Build history of the part. All positions in model axes, mm. A direction names the side the tool comes from. Give positions to 0.01 mm unless a question says otherwise; leave off trailing zeros. Order: outer loops, then holes, each group sorted by start corner. A loop starts at its lowest first (then second) coordinate and runs counter-clockwise, first axis right, second up. Notation, with made-up numbers: (-27, -19) - (30, -19) arc R25 ccw to (30, 20) - close; hole circle Ø5 at (23, 38). An arc over 180 degrees is marked (long way). Answer in a Markdown table with one row per item.
```python
from build123d import *

# Parameters (mm, degrees)
SKETCH1_R           = 18.25
BOSS_EXTRUDE1_DEPTH = 57
SKETCH2_R           = 6.5
BOSS_EXTRUDE2_DEPTH = 5
FILLET1_R           = 1.5
SKETCH3_R           = 1.6
BOSS_EXTRUDE3_DEPTH = 8.5
BOSS_EXTRUDE4_START = -2.5
SKETCH4_R           = 3.9
BOSS_EXTRUDE4_DEPTH = 5
SKETCH5_R           = 5
BOSS_EXTRUDE5_DEPTH = 3
SKETCH6_R           = 1.5
BOSS_EXTRUDE6_DEPTH = 2
SKETCH7_W           = 0.5
SKETCH7_H           = 5
BOSS_EXTRUDE7_DEPTH = 10
CHAMFER1_SIZE       = 1


with BuildPart() as part:
    # Sketch1 → Boss-Extrude1 (new body)
    with BuildSketch(Plane(origin=(0, 0, 0), x_dir=(1, 0, 0), z_dir=(0, 1, 0))):
        Circle(SKETCH1_R)
    extrude(amount=BOSS_EXTRUDE1_DEPTH)

    # Sketch2 → Boss-Extrude2 (add)
    with BuildSketch(Plane(origin=(0, 57, 0), x_dir=(1, 0, 0), z_dir=(0, 1, 0))):
        Circle(SKETCH2_R)
    extrude(amount=BOSS_EXTRUDE2_DEPTH)

    # Fillet1
    fillet1_edges = [part.edges().sort_by_distance(p)[0] for p in [
        (-18.25, 57, 0),
    ]]
    fillet(fillet1_edges, radius=FILLET1_R)

    # Sketch3 → Boss-Extrude3 (add)
    with BuildSketch(Plane(origin=(0, 62, 0), x_dir=(1, 0, 0), z_dir=(0, 1, 0))):
        Circle(SKETCH3_R)
    extrude(amount=BOSS_EXTRUDE3_DEPTH)

    # Sketch4 → Boss-Extrude4 (add)
    with BuildSketch(Plane(origin=(0, 70.5, 0), x_dir=(1, 0, 0), z_dir=(0, 1, 0)).offset(BOSS_EXTRUDE4_START)):
        Circle(SKETCH4_R)
    extrude(amount=-BOSS_EXTRUDE4_DEPTH)

    # Sketch5 → Boss-Extrude5 (add)
    with BuildSketch(Plane.XZ):
        Circle(SKETCH5_R)
    extrude(amount=BOSS_EXTRUDE5_DEPTH)

    # Sketch6 → Boss-Extrude6 (add)
    with BuildSketch(Plane.XZ.offset(3)):
        Circle(SKETCH6_R)
    extrude(amount=BOSS_EXTRUDE6_DEPTH)

    # Sketch7 → Boss-Extrude7 (add)
    with BuildSketch(Plane.XZ):
        with Locations((15.2, 0)):
            Rectangle(SKETCH7_W, SKETCH7_H)
        with Locations((-15.2, 0)):
            Rectangle(SKETCH7_W, SKETCH7_H)
    extrude(amount=BOSS_EXTRUDE7_DEPTH)

    # Chamfer1
    chamfer1_edges = [part.edges().sort_by_distance(p)[0] for p in [
        (15.2, -10, -2.5),
        (15.2, -10, 2.5),
        (-15.2, -10, -2.5),
        (-15.2, -10, 2.5),
    ]]
    chamfer(chamfer1_edges, length=CHAMFER1_SIZE)


solid = part.part
```
1. Cut at B-B on y = 50.5. Write the cut outline in (x, z), and give its area (3 significant figures).
Check result:
| item | result |
|---|---|
| outline | circle Ø36.5 at (0, 0) |
| area | 1,050 mm² |
2. Probe line 1 (Y direction, x = -12.5, z = 7.5); line 2 (Y direction, x = 6, z = 2); line 3 (Z direction, x = 7, y = 35.5). List the from-to ranges inside material, lowest first.
Check result:
| item | result |
|---|---|
| line 1 | y = 0 to 57 |
| line 2 | y = 0 to 62 |
| line 3 | z = -16.85 to 16.85 |
3. Drop flat-ended pins along their axis: P1, Ø1, axis at x = -1.5, y = 7, coming from the -Z side; P2, Ø1.5, axis at y = -3, z = 0.5, coming from the -X side; P3, Ø4, axis at x = 3.5, z = 13.5, coming from the +Y side. Give the stop position or say it passes through.
Check result:
| item | result |
|---|---|
| P1 | stops at z = -18.22 |
| P2 | stops at x = -15.45 |
| P3 | stops at y = 57 |
4. Two-plate mould, pull along Y, no slides. Class faces 1 (the face through (2, 63, 0)), 2 (the face through (-1.08, -1.48, -4.88)), 3 (the face through (0, 57, 7)): +Y half, -Y half, draft (parallel to the pull), parting line (faces both ways), or undercut.
Check result:
| item | result |
|---|---|
| face 1 | undercut |
| face 2 | draft |
| face 3 | +Y half |
5. Which spindle directions (+Z, -Z, +X, -X, +Y, -Y) get a long thin tool onto all of the face, cutting with end or side? Do faces 4 (the face through (-14.95, -5, 0)), 5 (the face through (4, 0, 4)), 6 (the face through (15.45, -5, 0)), 7 (the face through (1.4, 62, 1.4)), 8 (the face through (-2.87, 65.54, -2.64)). Say none if no direction does.
Check result:
| item | result |
|---|---|
| face 4 | +Z, -Z, -Y |
| face 5 | -Y |
| face 6 | +Z, -Z, +X, -Y |
| face 7 | none |
| face 8 | +Y |
